from build123d import *

# Parameters (mm, degrees)
F1_DEPTH  = 6.35
F2_W      = 50.8
F2_H      = 101.6
F3_DEPTH  = 9.525
F4_W      = 50.8
F4_H      = 9.525
F5_DEPTH  = 76.2
F6_W      = 50.8
F6_H      = 9.525
F7_DEPTH  = 92.075
F8_R      = 6.35
F9_DEPTH  = 25.4
F10_W     = 50.8
F10_H     = 66.675
F10_H_2   = 50.8
F11_DEPTH = 9.525


with BuildPart() as f1:
    # F0 (on Top) → F1 (new body)
    with BuildSketch(Plane.XY):
        Polygon((-317.5, -330.2), (317.5, -330.2), (317.5, 228.6), (139.7, 228.6), (139.7, 330.2), (-317.5, 330.2), align=None)
    extrude(amount=F1_DEPTH)

    # F2 (on face) → F3 (join)
    with BuildSketch(Plane.XY.offset(6.35)):
        with Locations((-266.7, 279.4)):
            Rectangle(F2_W, F2_H)
        with Locations((-266.7, 381)):
            Rectangle(F2_W, F2_H)
    extrude(amount=F3_DEPTH)

    # F4 (on face) → F5 (join)
    with BuildSketch(Plane(origin=(0, 0, 0), x_dir=(1, 0, 0), z_dir=(0, 0, -1))):
        with Locations((38.1, -300.0375)):
            Rectangle(F4_W, F4_H)
    extrude(amount=F5_DEPTH)

    # F6 (on face) → F7 (join)
    with BuildSketch(Plane(origin=(0, 304.8, 0), x_dir=(-1, 0, 0), z_dir=(0, 1, 0))):
        with Locations((-38.1, -71.4375)):
            Rectangle(F6_W, F6_H)
    extrude(amount=F7_DEPTH)

    # F8 (on face) → F9 (cut)
    with BuildSketch(Plane(origin=(0, 0, -76.2), x_dir=(1, 0, 0), z_dir=(0, 0, -1))):
        with Locations((38.1, -384.175)):
            Circle(F8_R)
    extrude(amount=-F9_DEPTH, mode=Mode.SUBTRACT)

    # F10 (on face) → F11 (join)
    with BuildSketch(Plane.XY.offset(6.35)):
        with Locations((38.1, 363.5375)):
            Rectangle(F10_W, F10_H)
        with Locations((38.1, 304.8)):
            Rectangle(F10_W, F10_H_2)
    extrude(amount=F11_DEPTH)


solid = f1.part
Verification items for the finished model (mm, model axes). A direction names the side the tool comes from. Coordinates: 2 decimals unless noted, no trailing zeros. Write each loop counter-clockwise with the first axis right and the second up, starting at its lowest first coordinate (ties: lowest second). Pieces come first, ordered by that corner, then holes. Notation, with made-up numbers: M -30.75,49 L -16.75,49 A15 cw -16.75,60 Z; hole C -32.75,83 d11. An arc over 180 degrees is marked long. Use CSV: the item, a comma, the result in double quotes.
Q1. Set-up check for faces 4 (the flat face through (38, 295.275, -38)), 5 (the flat face through (-267, 382, 6.35)), 6 (the flat face through (38, 364, 6.35)): record each of +Z, -Z, +X, -X, +Y, -Y from which the full face is reachable in a straight line by a thin tool's end or side.
Computed values:
face 4,"-Z, +X, -X, -Y"
face 5,"-Z, +X, -X, +Y"
face 6,"+X, -X, +Y"
Q2. Mould release check, pull along Z, two halves, no side actions. Record for faces 1 (the flat face through (-267, 332, 15.875)), 2 (the flat face through (12.7, 323, -69)), 3 (the flat face through (38, 304.8, -33)): pulls with the +Z half, pulls with the -Z half, needs draft (parallel to the pull), parting line crosses it, or undercut.
Computed values:
face 1,"pulls with the +Z half"
face 2,"needs draft"
face 3,"undercut"
Q3. Thickness scan on line 1 along X through (y, z) = (351.5, 12); line 2 along Y through (x, z) = (38, -72) (3 decimals); line 3 along Z through (x, y) = (138.5, 191). Record the ranges inside material, lowest first. Write a range as [from, to].
Computed values:
line 1,"[-292.1, -241.3], [12.7, 63.5]"
line 2,"[295.275, 377.826], [390.524, 396.875]"
line 3,"[0, 6.35]"
Q4. Go/stop test with flat-tipped pins: P1, Ø15, axis at x = 33, z = -43.5, coming from the +Y side; P2, Ø10.5, axis at x = 41, z = 10.5, coming from the +Y side (3 decimals); P3, Ø6, axis at x = 168, y = 133, coming from the +Z side. Record where each tip stops, or that it passes through.
Computed values:
P1,"y = 304.8"
P2,"y = 396.875"
P3,"z = 6.35"
Q5. Section check B-B, the plane x = -103. Enter the section's corners in (y, z), and give its area (3 significant figures).
Computed values:
outline,"M -330.2,0 L 330.2,0 L 330.2,6.35 L -330.2,6.35 Z"
area,"4,190 mm²"
Q6. Section check A-A, the plane y = 177. Enter the section's corners in (x, z), and give its area (3 significant figures).
Computed values:
outline,"M -317.5,0 L 317.5,0 L 317.5,6.35 L -317.5,6.35 Z"
area,"4,030 mm²"
